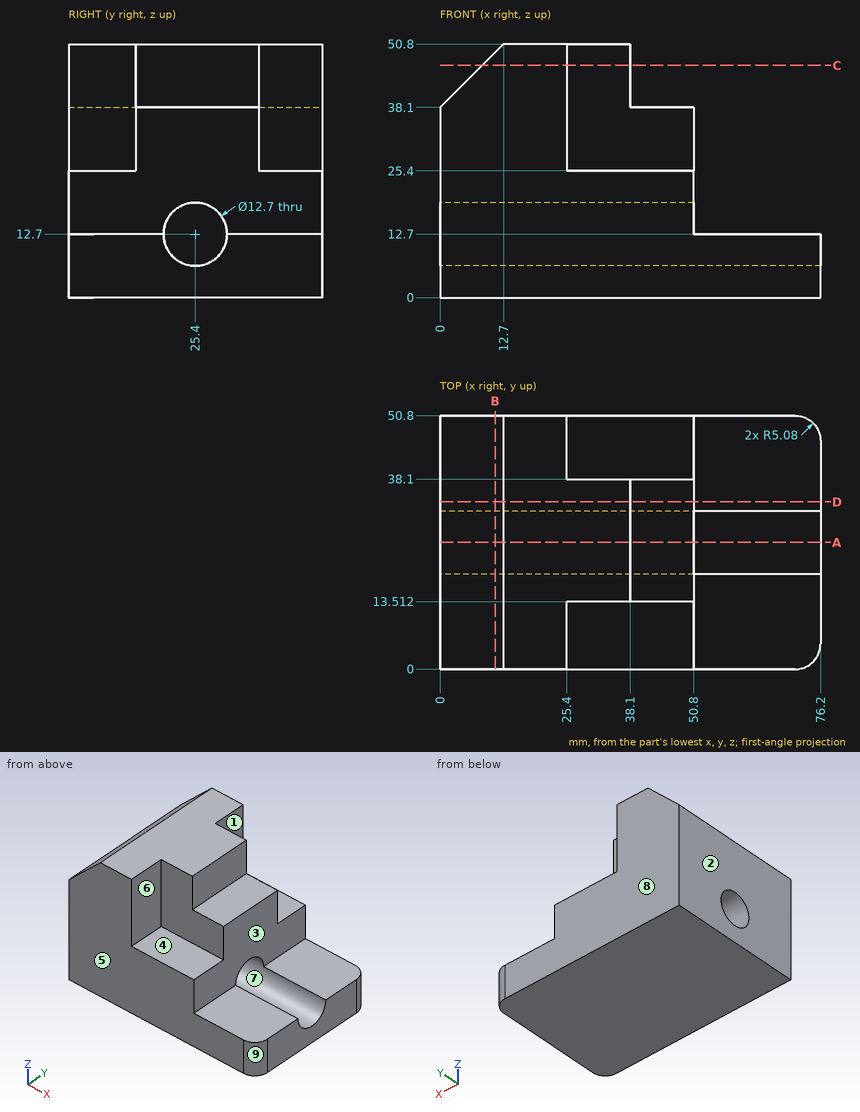
Design review of the part shown in the three views and the two pictorial views. Dimensions are in mm from the part's minimum x, y and z. A direction names the side the tool comes from. Round coordinates to 2 decimals unless told otherwise and drop trailing zeros. Loops run counter-clockwise (first coordinate to the right, second up) from the corner with the lowest first, then second, coordinate; pieces in that order, holes last.
Q1. Mouldability with a two-part tool opening along Y and no side actions: class the marked faces 6, 7, 8 and 9 as +Y half, -Y half, draft (parallel to the pull), parting line (faces both ways), or undercut.
Result sheet:
face 6: draft
face 7: undercut
face 8: +Y half
face 9: -Y half
Q2. Add section B-B on x = 11. Write out the cut boundary in (y, z).
Result sheet:
outline: (0, 0) - (50.8, 0) - (50.8, 49.1) - (0, 49.1) - close; hole circle Ø12.7 at (25.4, 12.7)
Q3. Machinability: for the marked faces 1, 2, 3, 4 and 5, which of the approach directions +Z, -Z, +X, -X, +Y, -Y give a long, thin tool a straight path to every point of the face, cutting with its end or side? Answer none if there is none.
Result sheet:
face 1: +Z, +X, +Y
face 2: +Z, -Z, -X, +Y, -Y
face 3: +Z, +X, +Y, -Y
face 4: +Z, +X, -Y
face 5: +Z, -Z, +X, -X, -Y
Q4. Add section C-C on z = 46.5. Write out the cut boundary in (x, y).
Result sheet:
outline: (8.4, 0) - (25.4, 0) - (25.4, 13.51) - (38.1, 13.51) - (38.1, 38.1) - (25.4, 38.1) - (25.4, 50.8) - (8.4, 50.8) - close
Q5. Add section D-D on y = 33.5. Write out the cut boundary in (x, z).
Result sheet:
outline: (0, 0) - (76.2, 0) - (76.2, 12.7) - (50.8, 12.7) - (50.8, 38.1) - (38.1, 38.1) - (38.1, 50.8) - (12.7, 50.8) - (0, 38.1) - close
Q6. Insertion check: pin 1 Ø7.5 at (x, z) = (41, 39.5) entering from -Y; pin 2 Ø15 at (x, y) = (62.5, 44) entering from +Z; pin 3 Ø4 at (y, z) = (30, 42) entering from +X. Each pin has a flat end and moves straight along its axis. Give the tip position at first contact, or say it passes through.
Result sheet:
pin 1: stops at y = 13.51
pin 2: stops at z = 12.7
pin 3: stops at x = 38.1
Q7. To check wall thickness, follow line 1 along Z through (x, y) = (47, 25); line 2 along Z through (x, y) = (21, 25.5); line 3 along Y through (x, z) = (19, 12.7). State the ranges of each line that lie inside material, in increasing order.
Result sheet:
line 1: z = 0 to 6.36, 19.04 to 38.1
line 2: z = 0 to 6.35, 19.05 to 50.8
line 3: y = 0 to 19.05, 31.75 to 50.8
Q8. Add section A-A on y = 25.4. Write out the cut boundary in (x, z).
Result sheet:
outline: (0, 0) - (76.2, 0) - (76.2, 6.35) - (0, 6.35) - close; (0, 19.05) - (50.8, 19.05) - (50.8, 38.1) - (38.1, 38.1) - (38.1, 50.8) - (12.7, 50.8) - (0, 38.1) - close
